```python
from build123d import *

# Parameters (mm, degrees)
BOSS_EXTRUDE1_DEPTH = 20
SKETCH2_R           = 5.25
CUT_EXTRUDE1_DEPTH  = 30
SKETCH3_R           = 3.125
CUT_EXTRUDE2_DEPTH  = 30
SKETCH4_R           = 5.25
CUT_EXTRUDE3_DEPTH  = 33
CHAMFER1_SIZE       = 2
SKETCH5_W           = 75
SKETCH5_H           = 20
CUT_EXTRUDE4_DEPTH  = 1.5


with BuildPart() as part:
    # Sketch1 → Boss-Extrude1 (new body)
    with BuildSketch(Plane.XY):
        with BuildLine():
            Line((-16, 0), (-37.5, 0))
            ThreePointArc((-37.5, 0), (0, -37.5), (37.5, 0))
            Line((37.5, 0), (16, 0))
            ThreePointArc((16, 0), (0, -16), (-16, 0))
        make_face()
    extrude(amount=BOSS_EXTRUDE1_DEPTH)

    # Sketch2 → Cut-Extrude1 (cut)
    with BuildSketch(Plane.XY.offset(20)):
        with Locations((-16.75187969, -23.05698434)):
            Circle(SKETCH2_R)
        with Locations((16.75187969, -23.05698434)):
            Circle(SKETCH2_R)
    extrude(amount=-CUT_EXTRUDE1_DEPTH, mode=Mode.SUBTRACT)

    # Sketch3 → Cut-Extrude2 (cut)
    with BuildSketch(Plane(origin=(0, 0, 0), x_dir=(1, 0, 0), z_dir=(0, 1, 0))):
        with Locations(Location((-26.75, -10, 0), (0, 0, 270))):
            Circle(SKETCH3_R)
        with Locations(Location((26.75, -10, 0), (0, 0, 270))):
            Circle(SKETCH3_R)
    extrude(amount=-CUT_EXTRUDE2_DEPTH, mode=Mode.SUBTRACT)

    # Sketch4 → Cut-Extrude3 (cut)
    with BuildSketch(Plane(origin=(0, -38, 0), x_dir=(1, 0, 0), z_dir=(0, 1, 0))):
        with Locations(Location((-26.75, -10, 0), (0, 0, 90))):
            Circle(SKETCH4_R)
        with Locations(Location((26.75, -10, 0), (0, 0, 90))):
            Circle(SKETCH4_R)
    extrude(amount=CUT_EXTRUDE3_DEPTH, mode=Mode.SUBTRACT)

    # Chamfer1
    chamfer1_edges = [part.edges().sort_by_distance(p)[0] for p in [
        (0, -37.5, 20),
    ]]
    chamfer(chamfer1_edges, length=CHAMFER1_SIZE)

    # Sketch5 → Cut-Extrude4 (cut)
    with BuildSketch(Plane(origin=(0, 0, 0), x_dir=(1, 0, 0), z_dir=(0, 1, 0))):
        with Locations((0, -10)):
            Rectangle(SKETCH5_W, SKETCH5_H)
    extrude(amount=-CUT_EXTRUDE4_DEPTH, mode=Mode.SUBTRACT)


solid = part.part
```
Geometry: final body of the model. Coordinates: model frame, mm. A direction names the side the tool comes from. Coordinates: 2 decimals unless noted, no trailing zeros. Order: outer loops, then holes, each group sorted by start corner. A loop starts at its lowest first (then second) coordinate and runs counter-clockwise, first axis right, second up. Notation, with made-up numbers: (31.25, 9.5) - (74.25, 9.5) arc R19 ccw to (74.25, 29.5) - close; hole circle Ø8 at (1.25, 48). An arc over 180 degrees is marked (long way). Return JSON: item names as keys, results as strings. Group by question number.
1. Cut plane A-A (z = 9.75). Output: boundary loops of the cut face in (x, y), plus the area to 3 significant figures.
2. Cut plane B-B (x = 0). Output: boundary loops of the cut face in (y, z).
3. Set-up query: faces 1 (the face through (-0.76, -35.62, 19.87)), 2 (the face through (30.2, -5, 10.1)). Return all of +Z, -Z, +X, -X, +Y, -Y with unobstructed straight access to the full face (end or side cutting, diameter ignored); none if empty.
4. Pull-direction query (Z, two-part tool) for faces 3 (the face through (-11.744, -21.48, 10.14)), 4 (the face through (-23.65, -3.23, 9.59)), 5 (the face through (0, -18, 20)); classes: pulls with the +Z half, pulls with the -Z half, needs draft (parallel to the pull), parting line crosses it, or undercut.
5. Pin query (flat end, axial travel): pin 1 (1 mm diameter, centred on x = 3, z = 5.5, fed in from +Y); pin 2 (3 mm diameter, centred on y = -17, z = 4, fed in from +X); pin 3 (11.5 mm diameter, centred on x = -27, z = 8, fed in from -Y); pin 4 (9.5 mm diameter, centred on x = -16.75, y = -23.06, fed in from +Z). Return the tip coordinate at first contact, or that it passes through.
6. Cut plane D-D (z = 5.5). Output: boundary loops of the cut face in (x, y).
7. Material intervals for line 1 along Z through (x, y) = (27, -7); line 2 along X through (y, z) = (-2.95, 10) (3 decimals); line 3 along X through (y, z) = (-3, 8.25), sorted ascending. Write a range as [from, to].
8. Cut plane C-C (y = -3.5). Count the separate pieces of the cut face and the enclosed holes in it, plus the area to 3 significant figures.
Resolved:
{
 "1": {"outline": "(-37.47, -1.5) arc R37.5 ccw to (-31.99, -19.56) - (-31.99, -5) - (-29.86, -5) - (-29.86, -1.5) - close; (-23.64, -5) - (-21.51, -5) - (-21.51, -20.83) arc R5.25 cw (long way) to (-21.51, -25.28) - (-21.51, -30.72) arc R37.5 ccw to (21.51, -30.72) - (21.51, -25.28) arc R5.25 cw (long way) to (21.51, -20.83) - (21.51, -5) - (23.64, -5) - (23.64, -1.5) - (15.93, -1.5) arc R16 cw to (-15.93, -1.5) - (-23.64, -1.5) - close; (29.86, -5) - (31.99, -5) - (31.99, -19.56) arc R37.5 ccw to (37.47, -1.5) - (29.86, -1.5) - close", "area": "1,090 mm²"},
 "2": {"outline": "(-37.5, 0) - (-16, 0) - (-16, 20) - (-35.5, 20) - (-37.5, 18) - close"},
 "3": {"face 1": "+Z, -Y", "face 2": "-Y"},
 "4": {"face 3": "needs draft", "face 4": "undercut", "face 5": "pulls with the +Z half"},
 "5": {"pin 1": "stops at y = -15.61", "pin 2": "stops at x = 34.15", "pin 3": "stops at y = -30.9", "pin 4": "passes through"},
 "6": {"outline": "(-37.47, -1.5) arc R37.5 ccw to (-29.45, -23.21) - (-29.45, -5) - (-24.05, -5) - (-24.05, -28.78) arc R37.5 ccw to (24.05, -28.78) - (24.05, -5) - (29.45, -5) - (29.45, -23.21) arc R37.5 ccw to (37.47, -1.5) - (15.93, -1.5) arc R16 cw to (-15.93, -1.5) - close; hole circle Ø10.5 at (-16.75, -23.06); hole circle Ø10.5 at (16.75, -23.06)"},
 "7": {"line 1": "z = [0, 4.76], [15.24, 20]", "line 2": "x = [-37.384, -29.875], [-23.625, -15.726], [15.726, 23.625], [29.875, 37.384]", "line 3": "x = [-37.38, -29.34], [-24.16, -15.72], [15.72, 24.16], [29.34, 37.38]"},
 "8": {"separate pieces": "2", "enclosed holes": "2", "area": "804 mm²"}
}
